Read the model definition and answer for the solid it produces. Units are mm, in the model's axes. A direction names the side the tool comes from. Coordinates: 2 decimals unless noted, no trailing zeros. Loops run counter-clockwise (first coordinate to the right, second up) from the corner with the lowest first, then second, coordinate; pieces in that order, holes last. Notation, with made-up numbers: (-4, 1) -> (29, 1) arc R28 ccw to (29, 33) -> close; hole circle Ø3 at (76, 17.25). An arc over 180 degrees is marked (long way). One line per question, with ' | ' between items. Start each with the question number.
```python
from build123d import *

# Parameters (mm, degrees)
SKETCH_1_R        = 4.26
SKETCH_1_R_2      = 2.23
EXTRUDE_1_DEPTH   = 5.875
EXTRUDE_1_2_DEPTH = 5.875
EXTRUDE_START     = 5.875
SKETCH_2_R        = 3
EXTRUDE_2_DEPTH   = 2


with BuildPart() as part:
    # Sketch 1 → Extrude 1 (new, symmetric)
    with BuildSketch(Plane.XY):
        with Locations((-6.35, 0)):
            Circle(SKETCH_1_R)
        with Locations((-6.35, 0)):
            Circle(SKETCH_1_R_2, mode=Mode.SUBTRACT)
    extrude(amount=EXTRUDE_1_DEPTH, both=True)



with BuildPart() as body_2:
    # Sketch 1 → Extrude 1 2 (new, symmetric)
    with BuildSketch(Plane.XY):
        with Locations((6.35, 0)):
            Circle(SKETCH_1_R)
        with Locations((6.35, 0)):
            Circle(SKETCH_1_R_2, mode=Mode.SUBTRACT)
    extrude(amount=EXTRUDE_1_2_DEPTH, both=True)


with BuildPart() as part_1:
    add(part.part)

    add(body_2.part)  # Extrude 2 merges body 2
    # Sketch 2 → Extrude 2 (add)
    with BuildSketch(Plane.XY.offset(EXTRUDE_START)):
        with BuildLine():
            ThreePointArc((-4.232138826, 5.517496176), (-12.26, 0), (-4.232138826, -5.517496176))
            ThreePointArc((-4.232138826, -5.517496176), (0, -4.733152662), (4.232138826, -5.517496176))
            ThreePointArc((4.232138826, -5.517496176), (12.26, 0), (4.232138826, 5.517496176))
            ThreePointArc((4.232138826, 5.517496176), (0, 4.733152662), (-4.232138826, 5.517496176))
        make_face()
        with Locations((-6.35, 0)):
            Circle(SKETCH_2_R, mode=Mode.SUBTRACT)
        with Locations((6.35, 0)):
            Circle(SKETCH_2_R, mode=Mode.SUBTRACT)
    extrude_2 = extrude(amount=-EXTRUDE_2_DEPTH)

    # Mirror 1: Extrude 2 across plane
    add(extrude_2.mirror(Plane.XY))


solid = part_1.part
```
(1) A tool of negligible diameter and unlimited length cuts with its end or side. For faces 5 (the cylindrical face through (-12.258, 0.16, -4.889)), 6 (the flat face through (0, 0, 3.875)), from which of +Z, -Z, +X, -X, +Y, -Y can it reach the whole face along a straight path? Write none if from no direction.
(2) Determine the mould class of faces 1 (the cylindrical face through (4.58, -1.357, -0.082)), 2 (the flat face through (0, 0, -3.875)), 3 (the cylindrical face through (-0.061, -4.733, 4.889)), 4 (the cylindrical face through (12.258, -0.16, 4.889)) for opening direction Y: +Y half, -Y half, draft (parallel to the pull), parting line (faces both ways), or undercut.
(3) Section B-B on y = 0 is taken. Write down the section's boundary in (x, z) (3 decimals).
(4) Section C-C on z = -0.75 is taken. Write down the section's boundary in (x, y), plus the area to 3 significant figures.
(5) Find the intervals of material crossed by probe 1 along Y at (x, z) = (6.35, 3.25); probe 2 along Z at (x, y) = (1.5, 2.75) (3 decimals); probe 3 along X at (y, z) = (1.25, -1), in increasing order. Write a range as from..to.
(6) Section A-A on x = 6.35 is taken. Write down the section's boundary in (y, z) (3 decimals), plus the area to 3 significant figures.
(7) Each of these flat-tipped pins is pushed along its axis until it touches: pin 1 Ø1 at (x, z) = (0.5, 4.5) entering from -Y; pin 2 Ø2 at (y, z) = (4, -3.5) entering from +X; pin 3 Ø1 at (y, z) = (0.5, 3) entering from -X. Where does it stop, or does it pass through?
(8) Section D-D on y = 1.75 is taken. Write down the section's boundary in (x, z) (3 decimals).
Working result:
1) face 5: +Z, -Z | face 6: none
2) face 1: undercut | face 2: draft | face 3: -Y half | face 4: parting line
3) outline: (-12.26, -5.875) -> (-8.58, -5.875) -> (-8.58, 5.875) -> (-12.26, 5.875) -> (-12.26, 3.875) -> (-10.61, 3.875) -> (-10.61, -3.875) -> (-12.26, -3.875) -> close; (-4.12, -5.875) -> (4.12, -5.875) -> (4.12, 5.875) -> (-4.12, 5.875) -> close; (8.58, -5.875) -> (12.26, -5.875) -> (12.26, -3.875) -> (10.61, -3.875) -> (10.61, 3.875) -> (12.26, 3.875) -> (12.26, 5.875) -> (8.58, 5.875) -> close; hole (-2.09, -3.875) -> (2.09, -3.875) -> (2.09, 3.875) -> (-2.09, 3.875) -> close
4) outline: circle Ø8.52 at (-6.35, 0); circle Ø8.52 at (6.35, 0); hole circle Ø4.46 at (-6.35, 0); hole circle Ø4.46 at (6.35, 0) | area: 82.8 mm2
5) probe 1: y = -4.26..-2.23, 2.23..4.26 | probe 2: z = -5.875..-3.875, 3.875..5.875 | probe 3: x = -10.42..-8.2, -4.5..-2.28, 2.28..4.5, 8.2..10.42
6) outline: (-5.91, -5.875) -> (-2.23, -5.875) -> (-2.23, 5.875) -> (-5.91, 5.875) -> (-5.91, 3.875) -> (-4.26, 3.875) -> (-4.26, -3.875) -> (-5.91, -3.875) -> close; (2.23, -5.875) -> (5.91, -5.875) -> (5.91, -3.875) -> (4.26, -3.875) -> (4.26, 3.875) -> (5.91, 3.875) -> (5.91, 5.875) -> (2.23, 5.875) -> close | area: 60.9 mm2
7) pin 1: stops at y = -4.78 | pin 2: stops at x = 11.4 | pin 3: stops at x = -10.61
8) outline: (-11.995, -5.875) -> (-7.732, -5.875) -> (-7.732, 5.875) -> (-11.995, 5.875) -> (-11.995, 3.875) -> (-10.234, 3.875) -> (-10.234, -3.875) -> (-11.995, -3.875) -> close; (-4.968, -5.875) -> (4.968, -5.875) -> (4.968, 5.875) -> (-4.968, 5.875) -> close; (7.732, -5.875) -> (11.995, -5.875) -> (11.995, -3.875) -> (10.234, -3.875) -> (10.234, 3.875) -> (11.995, 3.875) -> (11.995, 5.875) -> (7.732, 5.875) -> close; hole (-2.466, -3.875) -> (2.466, -3.875) -> (2.466, 3.875) -> (-2.466, 3.875) -> close
